Geometry: final body of the model. Coordinates: model frame, mm. Face numbers are marked on the shaded views. A direction names the side the tool comes from. Coordinates: 2 decimals unless noted, no trailing zeros. One line per item, written item: value. Start each with the question number.
Item 1: Contact query for flat-ended pins moving along their axis: pin 1 Ø5 at (y, z) = (5, 9) entering from +X; pin 2 Ø3 at (y, z) = (12.5, 8.5) entering from +X; pin 3 Ø1 at (y, z) = (0, 6) entering from -X. Output: stop coordinate, or through.
Item 2: Set-up query: the marked faces 5 and 6. Return all of +Z, -Z, +X, -X, +Y, -Y with unobstructed straight access to the full face (end or side cutting, diameter ignored); none if empty.
Item 3: Mould query, pull axis Y, two halves, no side actions, for the marked faces 1, 2, 3 and 4. Classes: +Y half, -Y half, draft (parallel to the pull), parting line (faces both ways), or undercut.
Item 4: Ray query, probe 1 along Y at (x, z) = (-21.5, 3); probe 2 along Y at (x, z) = (-13, 9.5); probe 3 along X at (y, z) = (7, 4.25). Return the intervals inside material, ascending. Write a range as from..to.
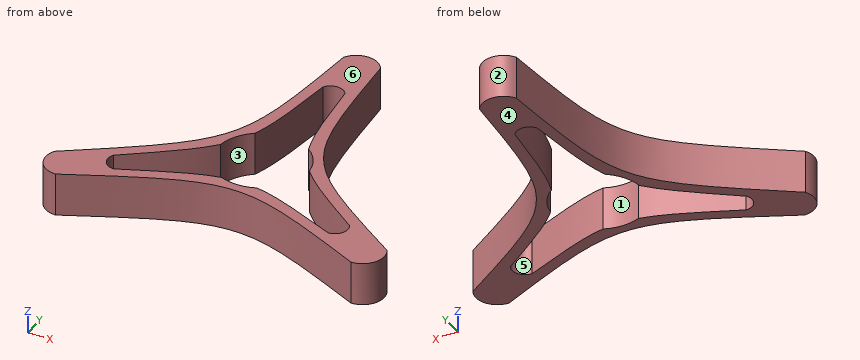
from build123d import *

# Parameters (mm, degrees)
F1_DEPTH = 10


with BuildPart() as f1:
    # F0 (on Top) → F1 (new body)
    with BuildSketch(Plane.XY):
        with BuildLine():
            add(Edge.make_bspline(
                [(4.330127, 42.5), (7.361216, 4.25), (7.361216, 4.25), (38.971143, -17.5)],
                knots=[0, 0, 0, 0, 69.282032, 69.282032, 69.282032, 69.282032], degree=3))
            ThreePointArc((4.330127, 42.5), (0, 45), (-4.330127, 42.5))
            add(Edge.make_bspline(
                [(-38.971143, -17.5), (-7.361216, 4.25), (-7.361216, 4.25), (-4.330127, 42.5)],
                knots=[0, 0, 0, 0, 69.282032, 69.282032, 69.282032, 69.282032], degree=3))
            ThreePointArc((-38.971143, -17.5), (-38.971143, -22.5), (-34.641016, -25))
            add(Edge.make_bspline(
                [(-34.641016, -25), (0, -8.5), (0, -8.5), (34.641016, -25)],
                knots=[0, 0, 0, 0, 69.282032, 69.282032, 69.282032, 69.282032], degree=3))
            ThreePointArc((34.641016, -25), (38.971143, -22.5), (38.971143, -17.5))
        make_face()
        with BuildLine():
            ThreePointArc((-10.429305, 1.216389), (-9.093267, 5.25), (-6.268076, 8.423848))
            add(Edge.make_bspline(
                [(-2.598076, 30.5), (-3.784006, 19.838289), (-4.505935, 13.348031), (-6.268076, 8.423848)],
                knots=[0, 0, 0, 0, 19.652555, 19.652555, 19.652555, 19.652555], degree=3))
            ThreePointArc((-2.598076, 30.5), (0, 32), (2.598076, 30.5))
            add(Edge.make_bspline(
                [(2.598076, 30.5), (3.784006, 19.838289), (4.505935, 13.34803), (6.268076, 8.423848)],
                knots=[0, 0, 0, 0, 19.652555, 19.652555, 19.652555, 19.652555], degree=3))
            ThreePointArc((6.268076, 8.423848), (9.093267, 5.25), (10.429305, 1.216389))
            add(Edge.make_bspline(
                [(10.429305, 1.216389), (13.812701, -2.771761), (19.072465, -6.642099), (27.712813, -13)],
                knots=[30.576918, 30.576918, 30.576918, 30.576918, 50.229473, 50.229473, 50.229473, 50.229473], degree=3))
            ThreePointArc((27.712813, -13), (27.712813, -16), (25.114737, -17.5))
            add(Edge.make_bspline(
                [(25.114737, -17.5), (15.288459, -13.19619), (9.306766, -10.576269), (4.161228, -9.640237)],
                knots=[0, 0, 0, 0, 19.652555, 19.652555, 19.652555, 19.652555], degree=3))
            ThreePointArc((4.161228, -9.640237), (0, -10.5), (-4.161228, -9.640237))
            add(Edge.make_bspline(
                [(-4.161228, -9.640237), (-9.306766, -10.576269), (-15.288459, -13.19619), (-25.114737, -17.5)],
                knots=[30.576918, 30.576918, 30.576918, 30.576918, 50.229473, 50.229473, 50.229473, 50.229473], degree=3))
            ThreePointArc((-25.114737, -17.5), (-27.712813, -16), (-27.712813, -13))
            add(Edge.make_bspline(
                [(-10.429305, 1.216389), (-13.812701, -2.771761), (-19.072465, -6.642099), (-27.712813, -13)],
                knots=[30.576918, 30.576918, 30.576918, 30.576918, 50.229473, 50.229473, 50.229473, 50.229473], degree=3))
        make_face(mode=Mode.SUBTRACT)
    extrude(amount=F1_DEPTH)


solid = f1.part
Reply:
1. pin 1: stops at x = 13.58
1. pin 2: stops at x = 8.77
1. pin 3: stops at x = -16.33
2. face 5: +Z, -Z
2. face 6: +Z, +X, -X, +Y, -Y
3. face 1: undercut
3. face 2: +Y half
3. face 3: undercut
3. face 4: draft
4. probe 1: y = -18.84..-15.92, -8.4..-5.01
4. probe 2: y = -15.32..-12.35, -1.47..3.23
4. probe 3: x = -10.55..-7.83, 7.83..10.55
